Autodesk Inventor part; units mm, degrees
ref_plane "YZ Plane" through (0, 0, 0) normal (1, 0, 0) x (0, 1, 0)
ref_plane "XZ Plane" through (0, 0, 0) normal (0, 1, 0) x (-1, 0, 0)
ref_plane "XY Plane" through (0, 0, 0) normal (0, 0, 1) x (1, 0, 0)
sketch "Sketch1" plane through (0, 0, 0) normal (0, 0, 1) x (1, 0, 0)
  line L0 (-90, -18) -> (90, -18)
  line L1 (90, -18) -> (90, 18)
  line L2 (90, 18) -> (-90, 18)
  line L3 (-90, 18) -> (-90, -18)
  line L4 (-90, -18) -> (90, 18) construction
  line L5 (90, -18) -> (-90, 18) construction
  line L6 (-46.05, 18) -> (46.05, 18)
  line L7 (46.05, 18) -> (46.05, 13)
  line L8 (46.05, 13) -> (-46.05, 13)
  line L9 (-46.05, 13) -> (-46.05, 18)
  line L10 (-46.05, 18) -> (46.05, 13) construction
  line L11 (46.05, 18) -> (-46.05, 13) construction
  line L12 (-90, -12.8) -> (-30, -12.8)
  line L13 (-30, -12.8) -> (-30, -18)
  line L14 (-30, -18) -> (-90, -18)
  line L15 (-90, -18) -> (-90, -12.8)
  line L16 (-90, -12.8) -> (-30, -18) construction
  line L17 (-30, -12.8) -> (-90, -18) construction
  line L18 (19.6182, -18) -> (70, -18)
  line L19 (0, 0) -> (0, -18) construction
  line L20 (30, -18) -> (90, -18)
  line L21 (90, -18) -> (90, -12.8)
  line L22 (90, -12.8) -> (30, -12.8)
  line L23 (30, -12.8) -> (30, -18)
  line L24 (30, -18) -> (90, -12.8) construction
  line L25 (90, -18) -> (30, -12.8) construction
  line L26 (-45.85, 18) -> (-74.05, 18)
  line L27 (74.05, 18) -> (74.05, 13)
  line L28 (74.05, 13) -> (90, 13)
  line L29 (-74.05, 18) -> (-74.05, 13)
  line L30 (-74.05, 13) -> (-90, 13)
  point P0 (0, 15.5)
  point P1 (-60, -15.4)
  point P2 (46.05, 18)
  point P3 (-46.05, 18)
  point P4 (-30, -18)
  point P5 (-90, -12.8)
  point P6 (60, -15.4)
  point P7 (30, -18)
  point P8 (-74.05, 18)
  dimension "d0" = 180
  dimension "d1" = 36
  dimension "d10" = 5
  dimension "d11" = 92.1
  dimension "d12" = 5.2
  dimension "d21" = 5.2
  dimension "d24" = 60
  dimension "d31" = 28
  dimension "d32" = 28
extrude "Extrusion1" add sketch "Sketch1" along normal blind 5 contours L13 L12 L3 L30 L29 L2 L9 L8 L7 L27 L28 L1 L22 L23 L0
equation "\"d32\" = d31"
properties part number "lower-front-back-plate-support"
The model under review builds one solid part; all positions refer to its coordinate system, in mm. A direction names the side the tool comes from. Coordinates: 2 decimals unless noted, no trailing zeros. Order: outer loops, then holes, each group sorted by start corner. A loop starts at its lowest first (then second) coordinate and runs counter-clockwise, first axis right, second up. Notation, with made-up numbers: (44, 37.25) -> (48, 37.25) arc R24 cw to (48, 58.25) -> close; hole circle Ø6 at (81.25, 55). An arc over 180 degrees is marked (long way). Answer in a Markdown table with one row per item. Add a question column.
Item 1: Mouldability with a two-part tool opening along X and no side actions: class faces 6 (the flat face through (-46.05, 15, 2)), 7 (the flat face through (1, 13, 2)), 8 (the flat face through (-82, 13, 2)), 9 (the flat face through (74.05, 16, 2)) as +X half, -X half, draft (parallel to the pull), parting line (faces both ways), or undercut.
Item 2: We need section B-B on x = -51.5. Write out the cut boundary in (y, z), plus the area to 3 significant figures.
Item 3: To check wall thickness, follow probe 1 along Y at (x, z) = (23.5, 4.55); probe 2 along Y at (x, z) = (-35.5, 1.6); probe 3 along X at (y, z) = (15, 1.25). State the ranges of each line that lie inside material, in increasing order.
Item 4: We need section C-C on x = -78. Write out the cut boundary in (y, z), plus the area to 3 significant figures.
Item 5: We need section A-A on z = 3.5. Write out the cut boundary in (x, y), plus the area to 3 significant figures.
Item 6: Machinability: for faces 1 (the flat face through (46.05, 16, 2)), 2 (the flat face through (-30, -15, 2)), 3 (the flat face through (-74.05, 16, 2)), 4 (the flat face through (82, 13, 2)), 5 (the flat face through (30, -15, 2)), which of the approach directions +Z, -Z, +X, -X, +Y, -Y give a long, thin tool a straight path to every point of the face, cutting with its end or side? Answer none if there is none.
Item 7: Clearance check with flat-ended pins moving along their axes: pin 1 (2.5 mm diameter, centred on x = 80, z = 3, fed in from +Y); pin 2 (1 mm diameter, centred on y = -14, z = 2, fed in from -X); pin 3 (1.5 mm diameter, centred on x = -55.5, z = 3, fed in from -Y). State where each tip first meets the part, or that it passes through.
Final values:
| question | item | result |
|---|---|---|
| 1 | face 6 | undercut |
| 1 | face 7 | undercut |
| 1 | face 8 | draft |
| 1 | face 9 | +X half |
| 2 | outline | (-12.8, 0) -> (18, 0) -> (18, 5) -> (-12.8, 5) -> close |
| 2 | area | 154 mm2 |
| 3 | probe 1 | y = -18 to 13 |
| 3 | probe 2 | y = -12.8 to 13 |
| 3 | probe 3 | x = -74.05 to -46.05, 46.05 to 74.05 |
| 4 | outline | (-12.8, 0) -> (13, 0) -> (13, 5) -> (-12.8, 5) -> close |
| 4 | area | 129 mm2 |
| 5 | outline | (-90, -12.8) -> (-30, -12.8) -> (-30, -18) -> (30, -18) -> (30, -12.8) -> (90, -12.8) -> (90, 13) -> (74.05, 13) -> (74.05, 18) -> (46.05, 18) -> (46.05, 13) -> (-46.05, 13) -> (-46.05, 18) -> (-74.05, 18) -> (-74.05, 13) -> (-90, 13) -> close |
| 5 | area | 5,240 mm2 |
| 6 | face 1 | +Z, -Z, +Y |
| 6 | face 2 | +Z, -Z, -X, -Y |
| 6 | face 3 | +Z, -Z, -X, +Y |
| 6 | face 4 | +Z, -Z, +X, +Y |
| 6 | face 5 | +Z, -Z, +X, -Y |
| 7 | pin 1 | stops at y = 13 |
| 7 | pin 2 | stops at x = -30 |
| 7 | pin 3 | stops at y = -12.8 |
